```python
from build123d import *

# Parameters (mm, degrees)
SKETCH1_R           = 3.5
BOSS_EXTRUDE1_DEPTH = 1.175
FILLET1_R           = 1
CHAMFER1_SIZE       = 0.2


with BuildPart() as part:
    # Sketch1 → Boss-Extrude1 (new body, symmetric)
    with BuildSketch(Plane(origin=(0, 0, 0), x_dir=(1, 0, 0), z_dir=(0, 1, 0))):
        Polygon((2.886751346, 5), (-2.886751346, 5), (-5.773502692, 0), (-2.886751346, -5), (2.886751346, -5), (5.773502692, 0), align=None)
        Circle(SKETCH1_R, mode=Mode.SUBTRACT)
    extrude(amount=BOSS_EXTRUDE1_DEPTH, both=True)

    # Fillet1
    fillet1_edges = [part.edges().sort_by_distance(p)[0] for p in [
        (5.773502692, 0, 0),
        (2.886751346, 0, 5),
        (-2.886751346, 0, 5),
        (-5.773502692, 0, 0),
        (-2.886751346, 0, -5),
        (2.886751346, 0, -5),
    ]]
    fillet(fillet1_edges, radius=FILLET1_R)

    # Chamfer1
    chamfer1_edges = [part.edges().sort_by_distance(p)[0] for p in [
        (-3.5, -1.175, 0),
        (-3.5, 1.175, 0),
        (4.330127019, -1.175, -2.5),
        (4.330127019, 1.175, -2.5),
        (4.330127019, -1.175, 2.5),
        (0, -1.175, 5),
        (-4.330127019, -1.175, 2.5),
        (-4.330127019, -1.175, -2.5),
        (0, -1.175, -5),
        (-2.809401077, -1.175, 4.866025404),
        (2.809401077, -1.175, -4.866025404),
        (-2.809401077, -1.175, -4.866025404),
        (-5.618802154, -1.175, 0),
        (2.809401077, -1.175, 4.866025404),
        (5.618802154, -1.175, 0),
        (4.330127019, 1.175, 2.5),
        (0, 1.175, -5),
        (-4.330127019, 1.175, -2.5),
        (-4.330127019, 1.175, 2.5),
        (0, 1.175, 5),
        (-2.809401077, 1.175, 4.866025404),
        (2.809401077, 1.175, -4.866025404),
        (-2.809401077, 1.175, -4.866025404),
        (-5.618802154, 1.175, 0),
        (2.809401077, 1.175, 4.866025404),
        (5.618802154, 1.175, 0),
    ]]
    chamfer(chamfer1_edges, length=CHAMFER1_SIZE)


solid = part.part
```
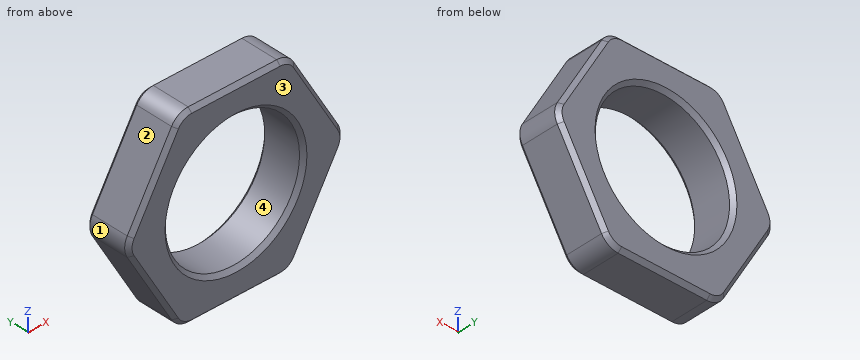
Part model, mm, in its own coordinate system. Face numbers are marked on the shaded views. Give positions to 0.01 mm unless a question says otherwise; leave off trailing zeros. Loops run counter-clockwise (first coordinate to the right, second up) from the corner with the lowest first, then second, coordinate; pieces in that order, holes last. Notation, with made-up numbers: M 65,6.5 L 105,6.5 A21 ccw 105,43.5 Z; hole C -19,33.25 d1. An arc over 180 degrees is marked long. Return JSON: item names as keys, results as strings.
1) Drill centre lines: line 1 (Z direction, x = 0, y = -0.2); line 2 (X direction, y = -0.45, z = 0); line 3 (Z direction, x = 2.5, y = -0.7). Where is each one in solid material? Low to high.
Calculated:
{"line 1": "z = -5 to -3.5, 3.5 to 5", "line 2": "x = -5.62 to -3.5, 3.5 to 5.62", "line 3": "z = -4.98 to -2.45, 2.45 to 4.98"}
2) Flat gauge pins, fed straight in: pin 1 Ø3 at (x, z) = (2, -2.5) entering from +Y (3 decimals); pin 2 Ø4 at (x, z) = (1, -0.5) entering from +Y. Where does each tip first touch, or does it go through?
Calculated:
{"pin 1": "stops at y = 1.175", "pin 2": "passes through"}
3) Saw through at B-B, the plane z = 0. List the corners of the cut face in (x, y) (3 decimals), then the cut area to 3 significant figures.
Calculated:
{"outline": "M -5.619,-0.975 L -5.419,-1.175 L -3.7,-1.175 L -3.5,-0.975 L -3.5,0.975 L -3.7,1.175 L -5.419,1.175 L -5.619,0.975 Z; M 3.5,-0.975 L 3.7,-1.175 L 5.419,-1.175 L 5.619,-0.975 L 5.619,0.975 L 5.419,1.175 L 3.7,1.175 L 3.5,0.975 Z", "area": "9.80 mm2"}
4) Saw through at A-A, the plane x = 0. List the corners of the cut face in (y, z) (3 decimals).
Calculated:
{"outline": "M -1.175,-4.8 L -0.975,-5 L 0.975,-5 L 1.175,-4.8 L 1.175,-3.7 L 0.975,-3.5 L -0.975,-3.5 L -1.175,-3.7 Z; M -1.175,3.7 L -0.975,3.5 L 0.975,3.5 L 1.175,3.7 L 1.175,4.8 L 0.975,5 L -0.975,5 L -1.175,4.8 Z"}
5) Pull direction Z, two halves, no side cores. Call the marked faces 1, 2, 3 and 4: released by +Z, released by -Z, zero draft, split by the parting line, or undercut.
Calculated:
{"face 1": "split by the parting line", "face 2": "released by +Z", "face 3": "zero draft", "face 4": "undercut"}
6) Saw through at D-D, the plane z = 4. List the corners of the cut face in (x, y) (3 decimals).
Calculated:
{"outline": "M -3.464,-0.975 L -3.233,-1.175 L 3.233,-1.175 L 3.464,-0.975 L 3.464,0.975 L 3.233,1.175 L -3.233,1.175 L -3.464,0.975 Z"}
7) Saw through at C-C, the plane y = 0.65. List the corners of the cut face in (x, z), then the cut area to 3 significant figures.
Calculated:
{"outline": "M -5.48,-0.5 L -3.18,-4.5 A1 ccw -2.31,-5 L 2.31,-5 A1 ccw 3.18,-4.5 L 5.48,-0.5 A1 ccw 5.48,0.5 L 3.18,4.5 A1 ccw 2.31,5 L -2.31,5 A1 ccw -3.18,4.5 L -5.48,0.5 A1 ccw Z; hole C 0,0 d7", "area": "47.8 mm2"}
